Build history of the part. All positions in model axes, mm. A direction names the side the tool comes from. Coordinates: 2 decimals unless noted, no trailing zeros. Write each loop counter-clockwise with the first axis right and the second up, starting at its lowest first coordinate (ties: lowest second). Pieces come first, ordered by that corner, then holes.
```python
from build123d import *

# Parameters (mm, degrees)
F0_R     = 3.2
F0_W     = 10.2
F0_H     = 12.2
F1_DEPTH = 7.8
F2_START = 0.8
F0_R_2   = 2.4
F2_DEPTH = 6.2
F0_R_3   = 1
F0_R_4   = 2
F3_DEPTH = 0.8


# Not quite as in the source:
# - a feature names something its author has since deleted; it is built from what else it names


with BuildPart() as f1:
    # F0 (on Top) → F1 (new body)
    with BuildSketch(Plane.XY):
        with BuildLine():
            Line((5.1, 7.7), (-9.1, 7.7))
            ThreePointArc((-9.1, 7.7), (-11.7162950904, 6.6162950904), (-12.8, 4))
            Line((-12.8, 4), (-12.8, -4))
            ThreePointArc((-12.8, -4), (-11.7162950904, -6.6162950904), (-9.1, -7.7))
            Line((-9.1, -7.7), (5.1, -7.7))
            ThreePointArc((5.1, -7.7), (6.2313708499, -7.2313708499), (6.7, -6.1))
            Line((6.7, -6.1), (6.7, 6.1))
            ThreePointArc((6.7, 6.1), (6.2313708499, 7.2313708499), (5.1, 7.7))
        make_face()
        with Locations((-9.1, -4)):
            Circle(F0_R, mode=Mode.SUBTRACT)
        with Locations((-9.1, 4)):
            Circle(F0_R, mode=Mode.SUBTRACT)
        Rectangle(F0_W, F0_H, mode=Mode.SUBTRACT)
    extrude(amount=F1_DEPTH)

    # F0 (on Top) → F2 (join)
    with BuildSketch(Plane.XY.offset(F2_START)):
        with Locations((-9.1, -4)):
            Circle(F0_R)
        with Locations((-9.1, -4)):
            Circle(F0_R_2, mode=Mode.SUBTRACT)
        with Locations((-9.1, 4)):
            Circle(F0_R)
        with Locations((-9.1, 4)):
            Circle(F0_R_2, mode=Mode.SUBTRACT)
    extrude(amount=F2_DEPTH)

    # F0 (on Top) → F3 (join)
    with BuildSketch(Plane.XY):
        Rectangle(F0_W, F0_H)
        with Locations((0, -4.5)):
            Circle(F0_R_3, mode=Mode.SUBTRACT)
        Circle(F0_R_4, mode=Mode.SUBTRACT)
        with Locations((0, 4.5)):
            Circle(F0_R_3, mode=Mode.SUBTRACT)
    extrude(amount=F3_DEPTH)


solid = f1.part
```
1. Saw through at B-B on y = 0. List the corners of the cut face in (x, z).
Computed values:
outline: (-12.8, 0) - (-2, 0) - (-2, 0.8) - (-5.1, 0.8) - (-5.1, 7.8) - (-12.8, 7.8) - close; (2, 0) - (6.7, 0) - (6.7, 7.8) - (5.1, 7.8) - (5.1, 0.8) - (2, 0.8) - close
2. Saw through at A-A on x = 0. List the corners of the cut face in (y, z), plus the area to 3 significant figures.
Computed values:
outline: (-7.7, 0) - (-5.5, 0) - (-5.5, 0.8) - (-6.1, 0.8) - (-6.1, 7.8) - (-7.7, 7.8) - close; (-3.5, 0) - (-2, 0) - (-2, 0.8) - (-3.5, 0.8) - close; (2, 0) - (3.5, 0) - (3.5, 0.8) - (2, 0.8) - close; (5.5, 0) - (7.7, 0) - (7.7, 7.8) - (6.1, 7.8) - (6.1, 0.8) - (5.5, 0.8) - close
area: 28.3 mm2
3. Flat gauge pin, fed straight in: pin 1 (2 mm diameter, centred on x = -1.5, y = -3, fed in from +Z). Where does the tip first touch, or does it go through?
Computed values:
pin 1: stops at z = 0.8
4. Probe line 1 along Y through (x, z) = (0, 0.5); line 2 along Y through (x, z) = (-9.1, 7.5); line 3 along Y through (x, z) = (-9.1, 3.75). List the from-to ranges inside material, lowest first.
Computed values:
line 1: y = -7.7 to -5.5, -3.5 to -2, 2 to 3.5, 5.5 to 7.7
line 2: y = -7.7 to -7.2, -0.8 to 0.8, 7.2 to 7.7
line 3: y = -7.7 to -6.4, -1.6 to 1.6, 6.4 to 7.7
5. 3-axis set-ups, long thin cutter, end or side, ignore diameter. For faces 1 (the face through (5.1, 0, 4)), 2 (the face through (-12.8, 0, 4)), 3 (the face through (-6.048, 4.961, 0.394)): which of +Z, -Z, +X, -X, +Y, -Y reach the whole face in a straight line?
Computed values:
face 1: +Z
face 2: +Z, -Z, -X, +Y, -Y
face 3: -Z
6. Mould opens along X. For faces 4 (the face through (-11.69, 6.64, 3.85)), 5 (the face through (-2, 7.7, 4)), 6 (the face through (-11.498, -3.894, 3.857)), 7 (the face through (6.7, 0, 4)) say: +X half, -X half, draft (parallel to the pull), parting line (faces both ways), or undercut.
Computed values:
face 4: -X half
face 5: draft
face 6: undercut
face 7: +X half
7. Saw through at D-D on x = -7.5. List the corners of the cut face in (y, z), plus the area to 3 significant figures.
Computed values:
outline: (-7.7, 0) - (-6.77, 0) - (-6.77, 0.8) - (-5.79, 0.8) - (-5.79, 7) - (-6.77, 7) - (-6.77, 7.8) - (-7.7, 7.8) - close; (-2.21, 0.8) - (-1.23, 0.8) - (-1.23, 0) - (1.23, 0) - (1.23, 0.8) - (2.21, 0.8) - (2.21, 7) - (1.23, 7) - (1.23, 7.8) - (-1.23, 7.8) - (-1.23, 7) - (-2.21, 7) - close; (5.79, 0.8) - (6.77, 0.8) - (6.77, 0) - (7.7, 0) - (7.7, 7.8) - (6.77, 7.8) - (6.77, 7) - (5.79, 7) - close
area: 58.0 mm2
8. Saw through at C-C on z = 3. List the corners of the cut face in (x, y), plus the area to 3 significant figures.
Computed values:
outline: (-12.8, -4) arc R3.7 ccw to (-9.1, -7.7) - (5.1, -7.7) arc R1.6 ccw to (6.7, -6.1) - (6.7, 6.1) arc R1.6 ccw to (5.1, 7.7) - (-9.1, 7.7) arc R3.7 ccw to (-12.8, 4) - close; hole circle Ø4.8 at (-9.1, -4); hole circle Ø4.8 at (-9.1, 4); hole (-5.1, -6.1) - (5.1, -6.1) - (5.1, 6.1) - (-5.1, 6.1) - close
area: 133 mm2
